Can you work these out from the model? Positions are in its coordinate system, mm. A direction names the side the tool comes from. Give positions to 0.01 mm unless a question says otherwise; leave off trailing zeros. Loops run counter-clockwise (first coordinate to the right, second up) from the corner with the lowest first, then second, coordinate; pieces in that order, holes last. Notation, with made-up numbers: M 64.25,39 L 80.25,39 A33 cw 80.25,68 Z; hole C 3,-14 d3. An arc over 180 degrees is marked long. Use CSV: the item, a comma, the result in double quotes.
from build123d import *

# Parameters (mm, degrees)
BOSS_EXTRUDE1_DEPTH = 170
CUT_EXTRUDE1_DEPTH  = 165
BOSS_EXTRUDE2_DEPTH = 35
BOSS_EXTRUDE3_DEPTH = 35


with BuildPart() as part:
    # Sketch1 → Boss-Extrude1 (new body)
    with BuildSketch(Plane.XY):
        Polygon((0, 0), (0, -15), (150, -15), (150, 10), align=None)
    extrude(amount=BOSS_EXTRUDE1_DEPTH)

    # Sketch2 → Cut-Extrude1 (cut)
    with BuildSketch(Plane.XY.offset(170)):
        Polygon((5, 0.333333333), (5, -12.6), (145, -11.8), (145, 9.666666667), align=None)
    extrude(amount=-CUT_EXTRUDE1_DEPTH, mode=Mode.SUBTRACT)

    # Sketch3 → Boss-Extrude2 (add)
    with BuildSketch(Plane.XY.offset(170)):
        Polygon((145, -11.8), (145, -15), (117, -15), (117, -11.96), align=None)
    extrude(amount=BOSS_EXTRUDE2_DEPTH)

    # Sketch4 → Boss-Extrude3 (add)
    with BuildSketch(Plane.XY.offset(170)):
        Polygon((89, -12.12), (89, -15), (61, -15), (61, -12.28), align=None)
        Polygon((5, -12.6), (5, -15), (33, -15), (33, -12.44), align=None)
    extrude(amount=BOSS_EXTRUDE3_DEPTH)


solid = part.part
Q1. I want a section at C-C, the plane z = 90. Please give me the cut outline in (x, y).
Model answer:
outline,"M 0,-15 L 150,-15 L 150,10 L 145,9.67 L 145,-11.8 L 5,-12.6 L 5,0.33 L 0,0 Z"
Q2. For faces 4 (the flat face through (150, -3, 84)), 5 (the flat face through (2, -7, 170)), 6 (the flat face through (145, -1, 89)), which set-ups out of +Z, -Z, +X, -X, +Y, -Y let a thin tool reach every point of the face, with its end or its side?
Model answer:
face 4,"+Z, -Z, +X, +Y, -Y"
face 5,"+Z, -X, +Y, -Y"
face 6,"+Z, +Y"
Q3. I want a section at A-A, the plane z = 180. Please give me the cut outline in (x, y).
Model answer:
outline,"M 5,-15 L 33,-15 L 33,-12.44 L 5,-12.6 Z; M 61,-15 L 89,-15 L 89,-12.12 L 61,-12.28 Z; M 117,-15 L 145,-15 L 145,-11.8 L 117,-11.96 Z"
Q4. I'm going to push flat-ended pins straight in: P1, Ø6, axis at x = 16, y = -1.5, coming from the +Z side; P2, Ø2.5, axis at y = -14, z = 186, coming from the -X side; P3, Ø2.5, axis at y = -13, z = 184, coming from the +X side. Where does each tip first touch, or does it pass through?
Model answer:
P1,"z = 5"
P2,"x = 5"
P3,"x = 145"
Q5. Please list where these lines run through material, in increasing order: L1, parallel to X at y = -13, z = 182; L2, parallel to X at y = -3.25, z = 49.5; L3, parallel to Z at x = 21.5, y = -2.75. Write a range as from..to.
Model answer:
L1,"5..33, 61..89, 117..145"
L2,"0..5, 145..150"
L3,"0..5"
Q6. I want a section at D-D, the plane x = 43. Please give me the cut outline in (y, z).
Model answer:
outline,"M -15,0 L 2.87,0 L 2.87,5 L -12.38,5 L -12.38,170 L -15,170 Z"
Q7. I want a section at B-B, the plane y = -2.75. Please give me the cut outline in (x, z).
Model answer:
outline,"M 0,0 L 150,0 L 150,170 L 145,170 L 145,5 L 5,5 L 5,170 L 0,170 Z"
Q8. If we mould it in two halves opening along X, with no side actions, what happens to faces 1 (the flat face through (5, -6, 89)), 2 (the flat face through (147, -2, 170)), 3 (the flat face through (0, -7, 84))? For each: released by +X, released by -X, zero draft, split by the parting line, or undercut.
Model answer:
face 1,"undercut"
face 2,"zero draft"
face 3,"released by -X"
